Can you work these out from the model? Positions are in its coordinate system, mm. Face numbers are marked on the shaded views. A direction names the side the tool comes from. Coordinates: 2 decimals unless noted, no trailing zeros. Loops run counter-clockwise (first coordinate to the right, second up) from the corner with the lowest first, then second, coordinate; pieces in that order, holes last. Notation, with made-up numbers: (63, 81) -> (94, 81) arc R15 cw to (94, 105) -> close; hole circle Ø4 at (-4, 82). An arc over 180 degrees is marked (long way). Use one line per item in the form item = value. Start each with the question number.
(1) Imagine slicing it at B-B (y = 5). List the corners of the cut face in (x, z) for me.
(2) Imagine slicing it at C-C (x = 15). List the corners of the cut face in (y, z) for me.
(3) Thinking about a two-plate mould opening in Y: for the marked faces 1, 2 and 3, which applies, released by +Y, released by -Y, zero draft, split by the parting line, or undercut?
(4) On a 3-axis mill with a long thin cutter (end or side, diameter ignored), from which of +Z, -Z, +X, -X, +Y, -Y can I reach the whole of each face in a straight line? I mean the marked faces 4, 5 and 6. Say none if no direction works.
(5) Imagine slicing it at D-D (y = 33). List the corners of the cut face in (x, z) for me, plus the area to 3 significant figures.
(6) Imagine slicing it at A-A (z = 6.25). List the corners of the cut face in (x, y) for me.
(7) I need wall thicknesses on line 1 (Y direction, x = 6.75, z = 6); line 2 (Y direction, x = 4.5, z = 7.5); line 3 (Z direction, x = 4.75, y = 41). Which ranges of each line are inside material? Lowest first, please. Write a range as [from, to].
(8) I'm going to push flat-ended pins straight in: pin 1 (1 mm diameter, centred on x = 15.5, y = 30.5, fed in from +Z); pin 2 (1.5 mm diameter, centred on x = 7, y = 26.5, fed in from +Z); pin 3 (0.6 mm diameter, centred on x = 12, z = 6, fed in from -Y). Where does each tip first touch, or does it pass through?
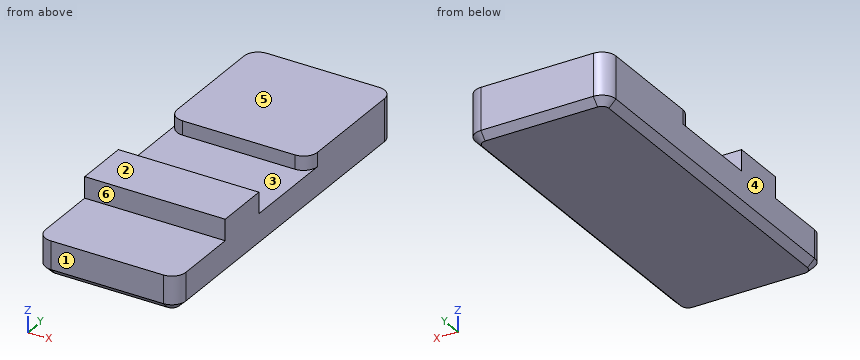
```python
from build123d import *

# Parameters (mm, degrees)
BOX_W        = 20
BOX_H        = 50
BOX_DEPTH    = 5
FILLET_R     = 2
CHAMFER_SIZE = 1
BOX001_W     = 20
BOX001_H     = 7.8
BOX001_DEPTH = 3
BOX002_W     = 20
BOX002_H     = 19.5
BOX002_DEPTH = 2
FILLET001_R  = 2


with BuildPart() as chamfer_body:
    # Box → Box (new body)
    with BuildSketch(Plane.XY):
        with Locations((10, 25)):
            Rectangle(BOX_W, BOX_H)
    extrude(amount=BOX_DEPTH)

    # Fillet
    fillet_edges = [chamfer_body.edges().sort_by_distance(p)[0] for p in [
        (0, 0, 2.5),
        (0, 50, 2.5),
        (20, 0, 2.5),
        (20, 50, 2.5),
    ]]
    fillet(fillet_edges, radius=FILLET_R)

    # Chamfer
    chamfer_edges = [chamfer_body.edges().sort_by_distance(p)[0] for p in [
        (0, 25, 0),
        (0.585786, 0.585786, 0),
        (0.585786, 49.414214, 0),
        (10, 0, 0),
        (19.414214, 0.585786, 0),
        (20, 25, 0),
        (19.414214, 49.414214, 0),
        (10, 50, 0),
    ]]
    chamfer(chamfer_edges, length=CHAMFER_SIZE)


with BuildPart() as cube001:
    # Box001 → Box001 (new body)
    with BuildSketch(Plane(origin=(0, 11.1, 5), x_dir=(1, 0, 0), z_dir=(0, 0, 1))):
        with Locations((10, 3.9)):
            Rectangle(BOX001_W, BOX001_H)
    extrude(amount=BOX001_DEPTH)


with BuildPart() as fusion:
    # Box002 → Box002 (new body)
    with BuildSketch(Plane(origin=(0, 30.5, 5), x_dir=(1, 0, 0), z_dir=(0, 0, 1))):
        with Locations((10, 9.75)):
            Rectangle(BOX002_W, BOX002_H)
    extrude(amount=BOX002_DEPTH)

    # Fillet001
    fillet001_edges = [fusion.edges().sort_by_distance(p)[0] for p in [
        (0, 30.5, 6),
        (0, 50, 6),
        (20, 30.5, 6),
        (20, 50, 6),
    ]]
    fillet(fillet001_edges, radius=FILLET001_R)

    # Fusion: union Chamfer body, Cube001
    add(chamfer_body.part)
    add(cube001.part)


solid = fusion.part
```
Worked out:
q1.outline = (0, 1) -> (1, 0) -> (19, 0) -> (20, 1) -> (20, 5) -> (0, 5) -> close
q2.outline = (0, 1) -> (1, 0) -> (49, 0) -> (50, 1) -> (50, 7) -> (30.5, 7) -> (30.5, 5) -> (18.9, 5) -> (18.9, 8) -> (11.1, 8) -> (11.1, 5) -> (0, 5) -> close
q3.face_1 = released by -Y
q3.face_2 = zero draft
q3.face_3 = undercut
q4.face_4 = +Z, -Z, -X, +Y, -Y
q4.face_5 = +Z, +X, -X, +Y
q4.face_6 = +Z, +X, -X, -Y
q5.outline = (0, 1) -> (1, 0) -> (19, 0) -> (20, 1) -> (20, 7) -> (0, 7) -> close
q5.area = 139 mm2
q6.outline = (0, 11.1) -> (20, 11.1) -> (20, 18.9) -> (0, 18.9) -> close; (0, 32.5) arc R2 ccw to (2, 30.5) -> (18, 30.5) arc R2 ccw to (20, 32.5) -> (20, 48) arc R2 ccw to (18, 50) -> (2, 50) arc R2 ccw to (0, 48) -> close
q7.line_1 = [11.1, 18.9], [30.5, 50]
q7.line_2 = [11.1, 18.9]
q7.line_3 = [0, 7]
q8.pin_1 = 7
q8.pin_2 = 5
q8.pin_3 = 11.1
